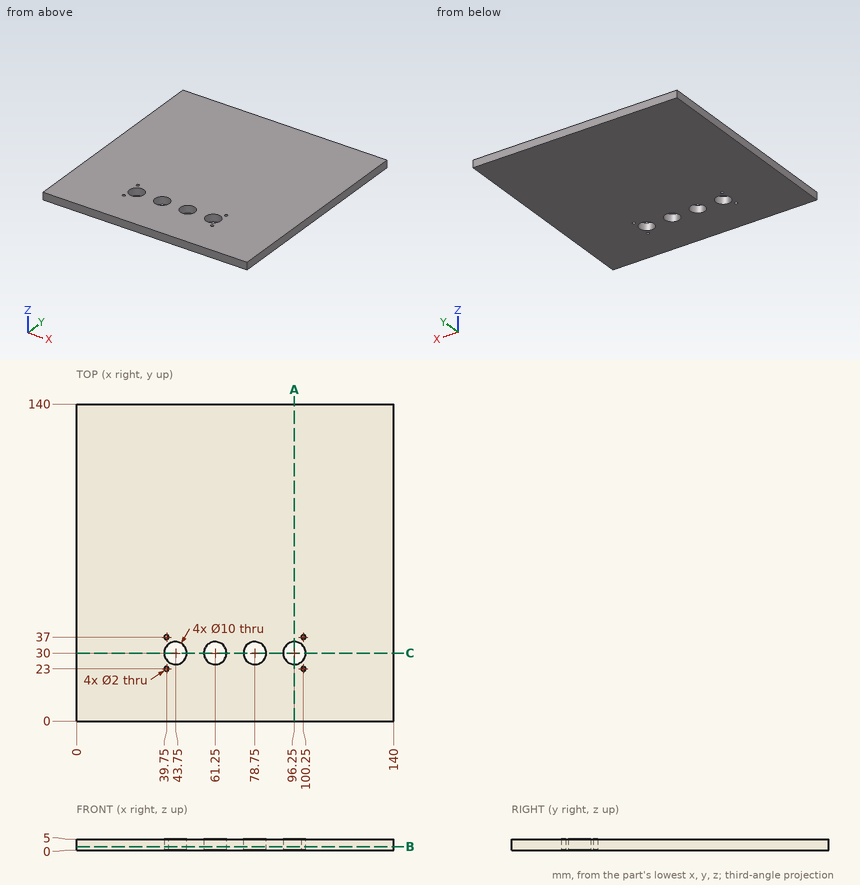
The figure shows three views and two pictorial views of one solid part (mm, origin at its lowest corner). Answer the questions. Give positions to 0.01 mm unless a question says otherwise; leave off trailing zeros. Write each loop counter-clockwise with the first axis right and the second up, starting at its lowest first coordinate (ties: lowest second). Pieces come first, ordered by that corner, then holes. Notation, with made-up numbers: (-40, 88) -> (-30, 88) arc R21 cw to (-30, 96) -> close; hole circle Ø5 at (32, -3.75). An arc over 180 degrees is marked (long way). Answer as a JSON object with one key per item and string values.
1) Straight lines are drawn through the part: probe 1 along X at (y, z) = (23, 1.35); probe 2 along Y at (x, z) = (43.75, 1.65); probe 3 along Y at (x, z) = (60.5, 1.3). For each, find the intervals that lie inside material, in ascending order. Write a range as from..to.
Findings below:
{"probe 1": "x = 0..38.75, 40.75..99.25, 101.25..140", "probe 2": "y = 0..25, 35..140", "probe 3": "y = 0..25.06, 34.94..140"}
2) Section B-B on z = 1.6 is taken. Count the separate pieces of the cut face and the enclosed holes in it, then the cut area to 3 significant figures.
Findings below:
{"separate pieces": "1", "enclosed holes": "8", "area": "19,300 mm^2"}
3) Section A-A on x = 96.25 is taken. Write down the section's boundary in (y, z).
Findings below:
{"outline": "(0, 0) -> (25, 0) -> (25, 5) -> (0, 5) -> close; (35, 0) -> (140, 0) -> (140, 5) -> (35, 5) -> close"}
4) A flat-ended cylindrical pin translates along its axis: pin 1 Ø1.6 at (x, y) = (100.25, 23) entering from +Z. Find the tip coordinate at first contact, or state that the pin passes through.
Findings below:
{"pin 1": "passes through"}
5) Section C-C on y = 30 is taken. Write down the section's boundary in (x, z).
Findings below:
{"outline": "(0, 0) -> (38.75, 0) -> (38.75, 5) -> (0, 5) -> close; (48.75, 0) -> (56.25, 0) -> (56.25, 5) -> (48.75, 5) -> close; (66.25, 0) -> (73.75, 0) -> (73.75, 5) -> (66.25, 5) -> close; (83.75, 0) -> (91.25, 0) -> (91.25, 5) -> (83.75, 5) -> close; (101.25, 0) -> (140, 0) -> (140, 5) -> (101.25, 5) -> close"}
